Can you work these out from the model? Positions are in its coordinate system, mm. Give positions to 0.01 mm unless a question says otherwise; leave off trailing zeros. Write each loop counter-clockwise with the first axis right and the second up, starting at its lowest first coordinate (ties: lowest second). Pieces come first, ordered by that corner, then holes.
1. I'm going to push a flat-ended pin straight in: pin 1 (2 mm diameter, centred on x = -130, y = 27, fed in from -Z). Where does the tip first touch, or does it pass through?
2. Thinking about a two-plate mould opening in X: for faces 1 (the cylindrical face through (-40.86, -69.68, 1.48)), 2 (the flat face through (-2, -3, 3)), which applies, pulls with the +X half, pulls with the -X half, needs draft (parallel to the pull), parting line crosses it, or undercut?
3. If I drill on probe 1 along X at (y, z) = (-71.5, 1.1); probe 2 along Y at (x, z) = (92.5, 0.85); probe 3 along X at (y, z) = (-54, 0.2), over which ranges is the centre line in solid material (lowest first)?
4. Suppose I cut it at A-A (x = -39.38). Please give me the cut outline in (y, z).
```python
from build123d import *

# Parameters (mm, degrees)
SKETCH_1_W          = 280
SKETCH_1_H          = 200
EXTRUDE_1_DEPTH     = 3
SKETCH_2_R          = 1.5
SKETCH_2_R_2        = 2.75
SKETCH_2_R_3        = 2.5
CUT_EXTRUDE_1_DEPTH = 3
SKETCH_3_W          = 280
SKETCH_3_H          = 8
CUT_EXTRUDE_2_DEPTH = 173.072659072
SKETCH_4_R          = 1.65
CUT_EXTRUDE_4_DEPTH = 173.072659072


with BuildPart() as part:
    # 草图1 → 凸台-拉伸1 (new body)
    with BuildSketch(Plane.XY):
        Rectangle(SKETCH_1_W, SKETCH_1_H)
    extrude(amount=EXTRUDE_1_DEPTH)

    # 草图2 → 切除-拉伸1 (cut)
    with BuildSketch(Plane(origin=(0, 0, 0), x_dir=(-1, 0, 0), z_dir=(0, 0, -1))):
        with Locations((92.5, 19.5)):
            Circle(SKETCH_2_R)
        with Locations((92.5, 35.5)):
            Circle(SKETCH_2_R)
        with Locations((92.5, 3.5)):
            Circle(SKETCH_2_R)
        with Locations((92.5, -28.5)):
            Circle(SKETCH_2_R)
        with Locations((92.5, 67.5)):
            Circle(SKETCH_2_R)
        with Locations((72.5, 67.5)):
            Circle(SKETCH_2_R)
        with Locations((72.5, 35.5)):
            Circle(SKETCH_2_R)
        with Locations((72.5, 19.5)):
            Circle(SKETCH_2_R)
        with Locations((72.5, 3.5)):
            Circle(SKETCH_2_R)
        with Locations((72.5, -28.5)):
            Circle(SKETCH_2_R)
        with Locations((-92.5, -28.5)):
            Circle(SKETCH_2_R)
        with Locations((-92.5, 3.5)):
            Circle(SKETCH_2_R)
        with Locations((-92.5, 19.5)):
            Circle(SKETCH_2_R)
        with Locations((-92.5, 35.5)):
            Circle(SKETCH_2_R)
        with Locations((-92.5, 67.5)):
            Circle(SKETCH_2_R)
        with Locations((-72.5, -28.5)):
            Circle(SKETCH_2_R)
        with Locations((-72.5, 3.5)):
            Circle(SKETCH_2_R)
        with Locations((-72.5, 19.5)):
            Circle(SKETCH_2_R)
        with Locations((-72.5, 35.5)):
            Circle(SKETCH_2_R)
        with Locations((-72.5, 67.5)):
            Circle(SKETCH_2_R)
        with Locations((39.38, -72)):
            Circle(SKETCH_2_R_2)
        with Locations((-6.62, -72)):
            Circle(SKETCH_2_R_2)
        with Locations((-2.5, -6.5)):
            Circle(SKETCH_2_R_3)
        with Locations((-32.5, -6.5)):
            Circle(SKETCH_2_R_3)
    extrude(amount=-CUT_EXTRUDE_1_DEPTH, mode=Mode.SUBTRACT)

    # 草图3 → 切除-拉伸2 (cut, through all)
    with BuildSketch(Plane(origin=(0, 0, 0), x_dir=(-1, 0, 0), z_dir=(0, 0, -1))):
        with Locations((0, 96)):
            Rectangle(SKETCH_3_W, SKETCH_3_H)
    extrude(amount=-CUT_EXTRUDE_2_DEPTH, mode=Mode.SUBTRACT)

    # 草图4 → 切除-拉伸4 (cut, through all)
    with BuildSketch(Plane(origin=(0, 0, 0), x_dir=(-1, 0, 0), z_dir=(0, 0, -1))):
        with Locations((-130, 75)):
            Circle(SKETCH_4_R)
        with Locations((-130, 59)):
            Circle(SKETCH_4_R)
        with Locations((-130, 43)):
            Circle(SKETCH_4_R)
        with Locations((-130, 27)):
            Circle(SKETCH_4_R)
        with Locations((-130, 11)):
            Circle(SKETCH_4_R)
        with Locations((-130, -5)):
            Circle(SKETCH_4_R)
        with Locations((-130, -21)):
            Circle(SKETCH_4_R)
        with Locations((-130, -37)):
            Circle(SKETCH_4_R)
        with Locations((-130, -53)):
            Circle(SKETCH_4_R)
        with Locations((-130, -69)):
            Circle(SKETCH_4_R)
        with Locations((-130, -85)):
            Circle(SKETCH_4_R)
        with Locations(Location((130, -85, 0), (0, 0, 180))):
            Circle(SKETCH_4_R)
        with Locations(Location((130, -69, 0), (0, 0, 180))):
            Circle(SKETCH_4_R)
        with Locations(Location((130, -53, 0), (0, 0, 180))):
            Circle(SKETCH_4_R)
        with Locations(Location((130, -37, 0), (0, 0, 180))):
            Circle(SKETCH_4_R)
        with Locations(Location((130, -21, 0), (0, 0, 180))):
            Circle(SKETCH_4_R)
        with Locations(Location((130, -5, 0), (0, 0, 180))):
            Circle(SKETCH_4_R)
        with Locations(Location((130, 11, 0), (0, 0, 180))):
            Circle(SKETCH_4_R)
        with Locations(Location((130, 27, 0), (0, 0, 180))):
            Circle(SKETCH_4_R)
        with Locations(Location((130, 43, 0), (0, 0, 180))):
            Circle(SKETCH_4_R)
        with Locations(Location((130, 59, 0), (0, 0, 180))):
            Circle(SKETCH_4_R)
        with Locations(Location((130, 75, 0), (0, 0, 180))):
            Circle(SKETCH_4_R)
    extrude(amount=-CUT_EXTRUDE_4_DEPTH, mode=Mode.SUBTRACT)


solid = part.part
```
Checks:
1. pin 1: passes through
2. face 1: undercut
2. face 2: needs draft
3. probe 1: x = -140 to -42.08, -36.68 to 3.92, 9.32 to 140
3. probe 2: y = -100 to -30, -27 to 2, 5 to 18, 21 to 34, 37 to 66, 69 to 92
3. probe 3: x = -140 to -131.31, -128.69 to 128.69, 131.31 to 140
4. outline: (-100, 0) - (-74.75, 0) - (-74.75, 3) - (-100, 3) - close; (-69.25, 0) - (92, 0) - (92, 3) - (-69.25, 3) - close
